Build history of the part. All positions in model axes, mm. Give positions to 0.01 mm unless a question says otherwise; leave off trailing zeros. Write each loop counter-clockwise with the first axis right and the second up, starting at its lowest first coordinate (ties: lowest second). Pieces come first, ordered by that corner, then holes. Notation, with made-up numbers: (-34, -8) - (-9, -8) arc R24 ccw to (-9, 14) - close; hole circle Ø9 at (7, 18). An arc over 180 degrees is marked (long way). Use one line per item in the form item = value. Start each with the question number.
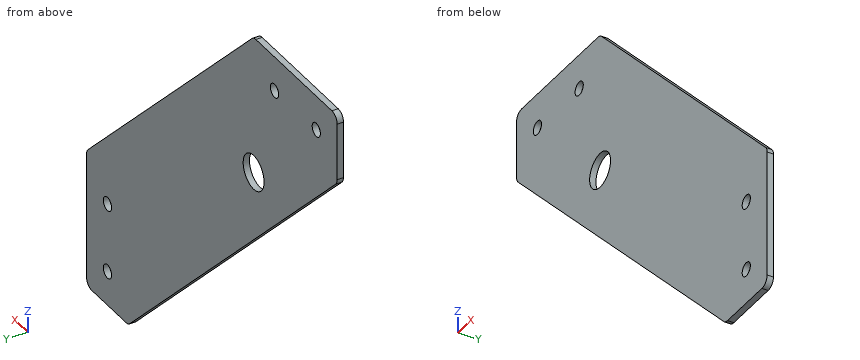
from build123d import *

# Parameters (mm, degrees)
SKETCH1_R           = 2.4892
SKETCH1_R_2         = 6.35
BOSS_EXTRUDE2_DEPTH = 1.143
CUT_EXTRUDE1_DEPTH  = 216.53826991
BOSS_EXTRUDE3_DEPTH = 2.286
FILLET3_R           = 3.175


with BuildPart() as part:
    # Sketch1 → Boss-Extrude2 (new, symmetric)
    with BuildSketch(Plane(origin=(0, 0, 0), x_dir=(1, 0, 0), z_dir=(0, 1, 0))):
        Polygon((0, 0), (0, 152.4), (-25.4, 152.4), (-152.4, 25.4), (-152.4, 0), align=None)
        with Locations(Location((-12.7, 12.7, 0), (0, 0, 270))):
            Circle(SKETCH1_R, mode=Mode.SUBTRACT)
        with Locations(Location((-38.1, 12.7, 0), (0, 0, 270))):
            Circle(SKETCH1_R, mode=Mode.SUBTRACT)
        with Locations(Location((-63.5, 12.7, 0), (0, 0, 270))):
            Circle(SKETCH1_R, mode=Mode.SUBTRACT)
        with Locations(Location((-88.9, 12.7, 0), (0, 0, 270))):
            Circle(SKETCH1_R, mode=Mode.SUBTRACT)
        with Locations(Location((-114.3, 12.7, 0), (0, 0, 270))):
            Circle(SKETCH1_R, mode=Mode.SUBTRACT)
        with Locations(Location((-12.7, 38.1, 0), (0, 0, 270))):
            Circle(SKETCH1_R, mode=Mode.SUBTRACT)
        with Locations(Location((-12.7, 63.5, 0), (0, 0, 270))):
            Circle(SKETCH1_R, mode=Mode.SUBTRACT)
        with Locations(Location((-12.7, 88.9, 0), (0, 0, 270))):
            Circle(SKETCH1_R, mode=Mode.SUBTRACT)
        with Locations(Location((-12.7, 114.3, 0), (0, 0, 270))):
            Circle(SKETCH1_R, mode=Mode.SUBTRACT)
        with Locations(Location((-139.7, 12.7, 0), (0, 0, 270))):
            Circle(SKETCH1_R, mode=Mode.SUBTRACT)
        with Locations(Location((-12.7, 139.7, 0), (0, 0, 270))):
            Circle(SKETCH1_R, mode=Mode.SUBTRACT)
        with Locations(Location((-101.6, 50.8, 0), (0, 0, 270))):
            Circle(SKETCH1_R_2, mode=Mode.SUBTRACT)
    extrude(amount=BOSS_EXTRUDE2_DEPTH, both=True)

    # Sketch2 → Cut-Extrude1 (cut, through all)
    with BuildSketch(Plane(origin=(0, 1.143, 0), x_dir=(1, 0, 0), z_dir=(0, 1, 0))):
        Polygon((0, 0), (0, 101.6), (-101.6, 0), align=None)
    extrude(amount=-CUT_EXTRUDE1_DEPTH, mode=Mode.SUBTRACT)

    # Sketch3 → Boss-Extrude3 (add)
    with BuildSketch(Plane(origin=(0, 1.143, 0), x_dir=(1, 0, 0), z_dir=(0, 1, 0))):
        Polygon((-101.6, 0), (-101.6, 15.120409187), (-15.612291765, 101.108117422), (0, 101.6), align=None)
    extrude(amount=-BOSS_EXTRUDE3_DEPTH)

    # Fillet3
    fillet3_edges = [part.edges().sort_by_distance(p)[0] for p in [
        (-101.6, 0, 0),
        (0, 0, -101.6),
        (-152.4, 0, 0),
        (-152.4, 0, -25.4),
        (-25.4, 0, -152.4),
        (0, 0, -152.4),
    ]]
    fillet(fillet3_edges, radius=FILLET3_R)


solid = part.part
(1) Cut at D-D, the plane y = 0.15. Give the cut face in (x, z) (3 decimals).
(2) Wall check: line 1 (X direction, y = 0.55, z = -12.7); line 2 (X direction, y = -0.6, z = -114.3); line 3 (Z direction, x = -139.7, y = 0). Give the ranges that are in metal, low to high. Write a range as from..to.
(3) Pin check, flat tip, straight feed: pin 1 Ø6.5 at (x, z) = (-12.7, -114.3) entering from +Y. Stop position of the tip, or through.
(4) Cut at A-A, the plane x = -12.7. Give the cut face in (y, z), then the cut area to 3 significant figures.
(5) Cut at B-B, the plane z = -114.3. Give the cut face in (x, y).
(6) Cut at C-C, the plane x = -114.3. Give the cut face in (y, z), then the cut area to 3 significant figures.
Solution:
q1.outline = (-152.4, -24.085) arc R3.175 ccw to (-151.47, -26.33) - (-26.33, -151.47) arc R3.175 ccw to (-24.085, -152.4) - (-3.175, -152.4) arc R3.175 ccw to (0, -149.225) - (0, -102.915) arc R3.175 ccw to (-0.93, -100.67) - (-100.67, -0.93) arc R3.175 ccw to (-102.915, 0) - (-149.225, 0) arc R3.175 ccw to (-152.4, -3.175) - close; hole circle Ø4.978 at (-139.7, -12.7); hole circle Ø4.978 at (-114.3, -12.7); hole circle Ø12.7 at (-101.6, -50.8); hole circle Ø4.978 at (-12.7, -139.7); hole circle Ø4.978 at (-12.7, -114.3)
q2.line_1 = -152.4..-142.19, -137.21..-116.79, -111.81..-88.9
q2.line_2 = -63.5..-15.19, -10.21..0
q2.line_3 = -38.1..-15.19, -10.21..0
q3.pin_1 = 1.14
q4.outline = (-1.14, -152.4) - (1.14, -152.4) - (1.14, -142.19) - (-1.14, -142.19) - close; (-1.14, -137.21) - (1.14, -137.21) - (1.14, -116.79) - (-1.14, -116.79) - close; (-1.14, -111.81) - (1.14, -111.81) - (1.14, -88.9) - (-1.14, -88.9) - close
q4.area = 122 mm2
q5.outline = (-63.5, -1.14) - (-15.19, -1.14) - (-15.19, 1.14) - (-63.5, 1.14) - close; (-10.21, -1.14) - (0, -1.14) - (0, 1.14) - (-10.21, 1.14) - close
q6.outline = (-1.14, -63.5) - (1.14, -63.5) - (1.14, -15.19) - (-1.14, -15.19) - close; (-1.14, -10.21) - (1.14, -10.21) - (1.14, 0) - (-1.14, 0) - close
q6.area = 134 mm2
